Can you work these out from the drawing? Everything is in mm from the part's minimum corner. Round coordinates to 2 decimals unless told otherwise and drop trailing zeros. Order: outer loops, then holes, each group sorted by start corner. A loop starts at its lowest first (then second) coordinate and runs counter-clockwise, first axis right, second up. Notation, with made-up numbers: M 29.5,61 L 47.5,61 A25 ccw 47.5,95 Z; hole C 40.25,-19.5 d11. An arc over 180 degrees is marked long. Answer as CSV lines item,"result". Start each with the question number.
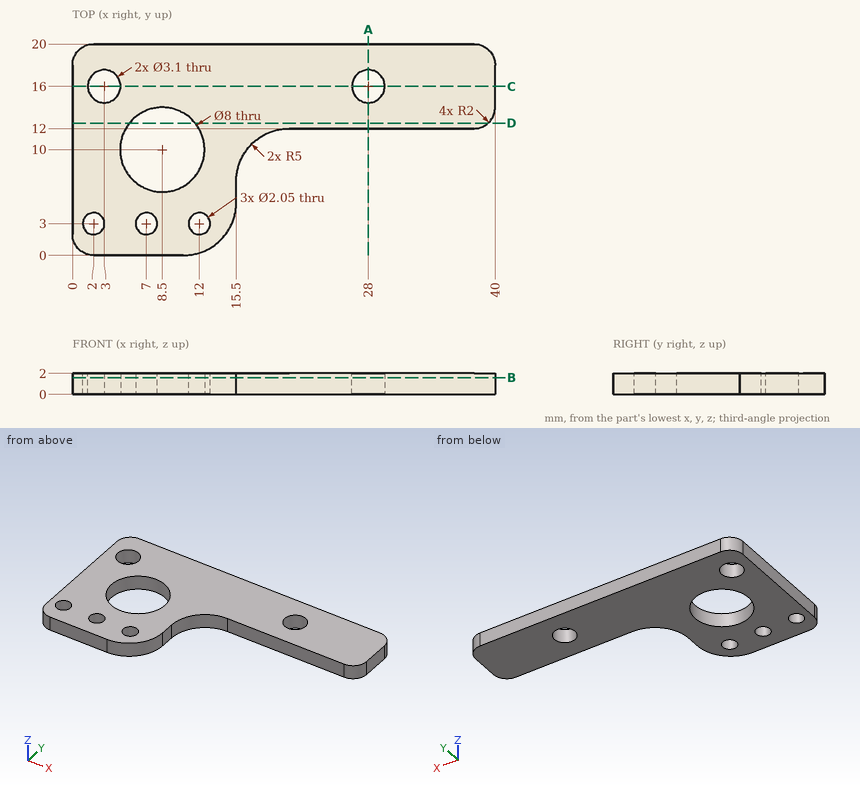
(1) I want a section at C-C on y = 16. Write out the boundary of the cut face in (x, z).
(2) I'm going to push flat-ended pins straight in: P1, Ø1.2, axis at x = 2, y = 3, coming from the -Z side; P2, Ø1, axis at x = 20.5, z = 1, coming from the -Y side (3 decimals). Where does each tip first touch, or does it pass through?
(3) If I drill on line 1 along Y through (x, z) = (28, 1.1); line 2 along X through (y, z) = (16.25, 1.85); line 3 along Y through (x, z) = (12, 1.5) (1 decimal), over which ranges is the centre line in solid material (lowest first)?
(4) I want a section at D-D on y = 12.5. Write out the boundary of the cut face in (x, z).
(5) I want a section at B-B on z = 1.6. Write out the boundary of the cut face in (x, y) (3 decimals), and give its area (3 significant figures).
(6) I want a section at A-A on x = 28. Write out the boundary of the cut face in (y, z).
From the geometry:
1,outline,"M 0,0 L 1.45,0 L 1.45,2 L 0,2 Z; M 4.55,0 L 26.45,0 L 26.45,2 L 4.55,2 Z; M 29.55,0 L 40,0 L 40,2 L 29.55,2 Z"
2,P1,"through"
2,P2,"y = 11.975"
3,line 1,"12 to 14.45, 17.55 to 20"
3,line 2,"0 to 1.47, 4.53 to 26.47, 29.53 to 40"
3,line 3,"0.2 to 2, 4 to 8.1, 11.9 to 20"
4,outline,"M 0,0 L 5.38,0 L 5.38,2 L 0,2 Z; M 11.62,0 L 39.32,0 L 39.32,2 L 11.62,2 Z"
5,outline,"M 0,2 A2 ccw 2,0 L 10.5,0 A5 ccw 15.5,5 L 15.5,7 A5 cw 20.5,12 L 38,12 A2 ccw 40,14 L 40,18 A2 ccw 38,20 L 2,20 A2 ccw 0,18 Z; hole C 2,3 d2.05; hole C 3,16 d3.1; hole C 8.5,10 d8; hole C 7,3 d2.05; hole C 12,3 d2.05; hole C 28,16 d3.1"
5,area,"427 mm²"
6,outline,"M 12,0 L 14.45,0 L 14.45,2 L 12,2 Z; M 17.55,0 L 20,0 L 20,2 L 17.55,2 Z"
